For this review, take the finished solid that the model builds, in its own axes (mm). Face numbers are marked on the shaded views. Round coordinates to 2 decimals unless told otherwise and drop trailing zeros. Write each loop counter-clockwise with the first axis right and the second up, starting at its lowest first coordinate (ties: lowest second). Pieces come first, ordered by that corner, then holes. Notation, with made-up numbers: M 42,54 L 96,54 A28 ccw 96,75 Z; hole C 0,38.25 d11. An arc over 180 degrees is marked long. Answer in a Markdown table with one row per item.
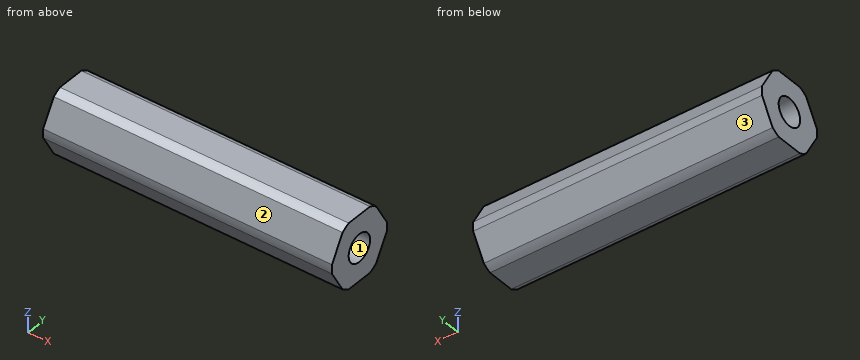
```python
from build123d import *

# Parameters (mm, degrees)
SKETCH1_R           = 2.667
BOSS_EXTRUDE1_DEPTH = 55.88


with BuildPart() as part:
    # Sketch1 → Boss-Extrude1 (new body)
    with BuildSketch(Plane(origin=(-41.275, 0, 0), x_dir=(0, -1, 0), z_dir=(-1, 0, 0))):
        with BuildLine():
            Line((4.175261692, -5.468234615), (6.823260936, -0.881765385))
            ThreePointArc((6.823260936, -0.881765385), (6.88, 0), (6.823260936, 0.881765385))
            Line((6.823260936, 0.881765385), (4.175261692, 5.468234615))
            ThreePointArc((4.175261692, 5.468234615), (3.44, 5.958254778), (2.647999245, 6.35))
            Line((2.647999245, 6.35), (-2.647999245, 6.35))
            ThreePointArc((-2.647999245, 6.35), (-3.44, 5.958254778), (-4.175261692, 5.468234615))
            Line((-4.175261692, 5.468234615), (-6.823260936, 0.881765385))
            ThreePointArc((-6.823260936, 0.881765385), (-6.88, 0), (-6.823260936, -0.881765385))
            Line((-6.823260936, -0.881765385), (-4.175261692, -5.468234615))
            ThreePointArc((-4.175261692, -5.468234615), (-3.44, -5.958254778), (-2.647999245, -6.35))
            Line((-2.647999245, -6.35), (2.647999245, -6.35))
            ThreePointArc((2.647999245, -6.35), (3.44, -5.958254778), (4.175261692, -5.468234615))
        make_face()
        with Locations(Location((0, 0, 0), (0, 0, 270))):
            Circle(SKETCH1_R, mode=Mode.SUBTRACT)
    extrude(amount=-BOSS_EXTRUDE1_DEPTH)


solid = part.part
```
Q1. Take a section at D-D (z = 4). State the section outline as (x, y) points (3 decimals), then the cut area to 3 significant figures.
Found:
| item | result |
|---|---|
| outline | M -41.275,-5.023 L 14.605,-5.023 L 14.605,5.023 L -41.275,5.023 Z |
| area | 561 mm² |
Q2. Take a section at C-C (y = 0). State the section outline as (x, z) points (3 decimals), then the cut area to 3 significant figures.
Found:
| item | result |
|---|---|
| outline | M -41.275,-6.35 L 14.605,-6.35 L 14.605,-2.667 L -41.275,-2.667 Z; M -41.275,2.667 L 14.605,2.667 L 14.605,6.35 L -41.275,6.35 Z |
| area | 412 mm² |
Q3. Insertion check: P1, Ø5, axis at x = -7, y = -3, coming from the -Z side; P2, Ø5, axis at x = -27, z = -4.5, coming from the -Y side; P3, Ø1.5, axis at x = -0.5, y = -4.5, coming from the +Z side. Each pin has a flat end and moves straight along its axis. Give the tip position at first contact, or say it passes through.
Found:
| item | result |
|---|---|
| P1 | z = -6.35 |
| P2 | y = -6.18 |
| P3 | z = 5.77 |
Q4. For probe 1 along Y at (x, z) = (-13.5, 0); probe 2 along Y at (x, z) = (4, 2); probe 3 along Z at (x, y) = (2.5, -3.5), list the stretches that pass through material, from the lowest coordinate up.
Found:
| item | result |
|---|---|
| probe 1 | -6.88 to -2.67, 2.67 to 6.88 |
| probe 2 | -6.18 to -1.76, 1.76 to 6.18 |
| probe 3 | -5.92 to 5.92 |
Q5. Take a section at A-A (z = 0). State the section outline as (x, y) points (3 decimals), then the cut area to 3 significant figures.
Found:
| item | result |
|---|---|
| outline | M -41.275,-6.88 L 14.605,-6.88 L 14.605,-2.667 L -41.275,-2.667 Z; M -41.275,2.667 L 14.605,2.667 L 14.605,6.88 L -41.275,6.88 Z |
| area | 471 mm² |
Q6. Take a section at B-B (x = 3). State the section outline as (y, z) points.
Found:
| item | result |
|---|---|
| outline | M -6.82,-0.88 L -4.18,-5.47 A6.88 ccw -2.65,-6.35 L 2.65,-6.35 A6.88 ccw 4.18,-5.47 L 6.82,-0.88 A6.88 ccw 6.82,0.88 L 4.18,5.47 A6.88 ccw 2.65,6.35 L -2.65,6.35 A6.88 ccw -4.18,5.47 L -6.82,0.88 A6.88 ccw Z; hole C 0,0 d5.33 |
Q7. Mouldability with a two-part tool opening along Z and no side actions: class the marked faces 1, 2 and 3 as +Z half, -Z half, draft (parallel to the pull), parting line (faces both ways), or undercut.
Found:
| item | result |
|---|---|
| face 1 | undercut |
| face 2 | +Z half |
| face 3 | -Z half |
